```python
from build123d import *

# Parameters (mm, degrees)
SWEEP1_PITCH        = 6.604
SWEEP1_HEIGHT       = 6.879166887
SWEEP1_RADIUS       = 15.875
SWEEP1_START_ANGLE  = -90
SKETCH4_R           = 2.38125
SKETCH5_R           = 2.38125
BOSS_EXTRUDE1_DEPTH = 15.24
SKETCH6_R           = 2.38125
BOSS_EXTRUDE2_DEPTH = 101.6
SKETCH7_R           = 2.38125
SKETCH13_W          = 34.723649491
SKETCH13_H          = 34.72364949
CUT_EXTRUDE1_DEPTH  = 76.2
SKETCH15_R          = 2.38125
BOSS_EXTRUDE5_DEPTH = 76.2


with BuildPart() as part:
    # Sweep1: sweep along a helix
    with BuildLine() as sweep1_path:
        add(Helix(SWEEP1_PITCH, SWEEP1_HEIGHT, SWEEP1_RADIUS, center=(0, 0, 0), direction=(0, 1, 0), lefthand=True, mode=Mode.PRIVATE).rotate(Axis((0, 0, 0), (0, 1, 0)), SWEEP1_START_ANGLE))
    # Sketch4 → Sweep1 (sweep)
    with BuildSketch(Plane.XY):
        with Locations((-15.875, 0)):
            Circle(SKETCH4_R)
    sweep(path=sweep1_path.line, is_frenet=True)

    # Sketch5 → Boss-Extrude1 (add)
    with BuildSketch(Plane(origin=(0, 0, 0), x_dir=(-0.965925772, 0, -0.258819247), z_dir=(0.258819247, 0, -0.965925772))):
        with Locations((15.875, 6.879489502)):
            Circle(SKETCH5_R)
    extrude(amount=BOSS_EXTRUDE1_DEPTH)

    # Sketch6 → Boss-Extrude2 (add)
    with BuildSketch(Plane.XY):
        with Locations((-15.875, 0)):
            Circle(SKETCH6_R)
    extrude(amount=BOSS_EXTRUDE2_DEPTH)

    # Sweep3: sweep along a path in Sketch8
    with BuildLine(Plane(origin=(-11.389666301, -1.880573246, 0), x_dir=(0, -1, 0), z_dir=(1, 0, 0))) as sweep3_path:
        ThreePointArc((-8.760062748, 18.829464319), (-10.247960299, 22.421566768), (-13.840062748, 23.909464319))
    # Sketch7 → Sweep3 (sweep)
    with BuildSketch(Plane(origin=(3.94440533, 0, -14.720708767), x_dir=(-0.965925772, 0, -0.258819247), z_dir=(0.258819247, 0, -0.965925772))):
        with Locations((15.875, 6.879489502)):
            Circle(SKETCH7_R)
    sweep(path=sweep3_path.line)

    # Sketch13 → Cut-Extrude1 (cut)
    with BuildSketch(Plane(origin=(0, 0, 0), x_dir=(0, 0, -1), z_dir=(1, 0, 0))):
        with Locations((15.752675198, 28.559314247)):
            Rectangle(SKETCH13_W, SKETCH13_H)
    extrude(amount=-CUT_EXTRUDE1_DEPTH, mode=Mode.SUBTRACT)

    # Sketch15 → Boss-Extrude5 (add)
    with BuildSketch(Plane(origin=(0, 11.197489502, 0), x_dir=(1, 0, 0), z_dir=(0, 1, 0))):
        with Locations((-11.372091381, 23.873869709)):
            Circle(SKETCH15_R)
    extrude(amount=BOSS_EXTRUDE5_DEPTH)


solid = part.part
```
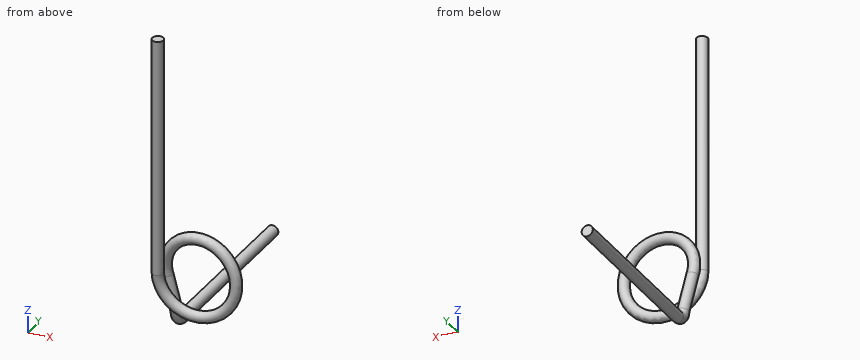
Could you check a few things on this model? Use its own coordinates, in mm. Round coordinates to 2 decimals unless told otherwise and drop trailing zeros. Loops run counter-clockwise (first coordinate to the right, second up) from the corner with the lowest first, then second, coordinate; pieces in that order, holes last. Notation, with made-up numbers: (80, 75.5) - (126, 75.5) arc R19 ccw to (126, 98.5) - close; hole circle Ø6 at (-33.5, 39.5). An arc over 180 degrees is marked (long way). Answer in a Markdown table with one row per item. Add a question column.
(1) I need wall thicknesses on line 1 along Y through (x, z) = (-14, 40.5); line 2 along Z through (x, y) = (1.5, 7); line 3 along Z through (x, y) = (-10, 32). Which ranges of each line are inside material? Lowest first, please.
(2) If we section it at A-A (z = 32.5): Please give me the cut outline in (x, y) (1 decimal), plus the area to 3 significant figures.
(3) If we section it at B-B (y = 45.5): Please give me the cut outline in (x, z).
(4) I'm going to push flat-ended pins straight in: pin 1 (10 mm diameter, centred on x = -10, z = 55.5, fed in from -Y); pin 2 (2 mm diameter, centred on x = -11.5, z = -23, fed in from -Y); pin 3 (10 mm diameter, centred on x = -9.5, z = -3.5, fed in from -Y). Where does each tip first touch, or does it pass through?
Model answer:
| question | item | result |
|---|---|---|
| 1 | line 1 | y = -1.47 to 1.47 |
| 1 | line 2 | z = 14.78 to 16.85 |
| 1 | line 3 | z = -25.82 to -21.93 |
| 2 | outline | circle Ø4.8 at (-15.9, 0) |
| 2 | area | 17.8 mm² |
| 3 | outline | circle Ø4.76 at (-11.37, -23.87) |
| 4 | pin 1 | stops at y = -2.21 |
| 4 | pin 2 | stops at y = 5.21 |
| 4 | pin 3 | stops at y = -1.94 |
